Solid Edge part; units mm, degrees
sketch "Sketch1" plane through (0, 0, 0) normal (0, -1, 0) x (1, 0, 0)
  line L0 (-5.8407, 6.1754) -> (-7.1398, 6.9254)
  line L1 (-7.1398, 6.9254) -> (-12.2436, -1.9148)
  line L2 (-12.2436, -1.9148) -> (-9.0862, -3.7377)
  line L3 (-9.0862, -3.7377) -> (-5.1962, 3)
  line L4 (6, 0) -> (6, -2.6279)
  line L5 (13.4768, -2.6279) -> (6, -2.6279)
  line L6 (13.4768, -0.6279) -> (13.4768, -2.6279)
  line L7 (8.4768, -0.6279) -> (13.4768, -0.6279)
  arc A0 (8.4768, -0.6279) -> (-5.8407, 6.1754) centre (0, 0) ccw
  arc A1 (-5.1962, 3) -> (6, 0) centre (0, 0) cw
  dimension "D1" = 5.8407
  dimension "D2" = 13.4768
  dimension "D3" = 8.4768
  dimension "D4" = 6
  dimension "D5" = 13.4768
  dimension "D6" = 12.2436
  dimension "D7" = 9.0862
  dimension "D8" = 7.1398
extrude "Protrusion1" add sketch "Sketch1" against normal blind 2
fillet "Round_1" radius 1 1 edges at (8.4768, 1, -0.6279)
fillet "Round_2" radius 0.5 1 edges at (6, 1, -2.6279)
fillet "Round_3" radius 2 1 edges at (-5.8407, 1, 6.1754)
fillet "Round_4" radius 0.5 1 edges at (-7.1398, 1, 6.9254)
hole "Hole___body" at (-9.6667, 0, -1.0932) direction (0, 1, 0) diameter 2 end up to next
fillet "Round_5" radius 1 2 edges at (-9.0862, 1, -3.7377) (-12.2436, 1, -1.9148)
properties material "ABS Plastic, high impact"
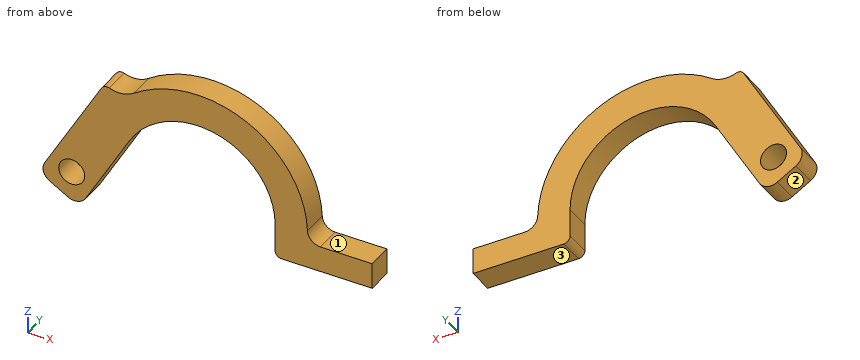
Build history of the part. All positions in model axes, mm. Face numbers are marked on the shaded views. A direction names the side the tool comes from. Round coordinates to 2 decimals unless told otherwise and drop trailing zeros. Loops run counter-clockwise (first coordinate to the right, second up) from the corner with the lowest first, then second, coordinate; pieces in that order, holes last. Notation, with made-up numbers: (-16.5, 64.5) -> (-5.5, 64.5) arc R10 ccw to (-5.5, 72.5) -> close; hole circle Ø4 at (86, -39.5). An arc over 180 degrees is marked (long way). Use CSV: the item, a comma, the result in double quotes. Start each with the question number.
Q1. Saw through at C-C on z = 7.5. Give the cut face in (x, y).
Q2. Which spindle directions (+Z, -Z, +X, -X, +Y, -Y) get a long thin tool onto all of the face, cutting with end or side? Do the marked faces 1, 2 and 3. Say none if no direction does.
Q3. Saw through at B-B on x = -9. Give the cut face in (y, z).
Q4. Saw through at A-A on z = 5.25. Give the cut face in (x, y).
Q5. Drill centre lines: L1, parallel to X at y = 0.9, z = -1; L2, parallel to X at y = 0.6, z = -2; L3, parallel to Z at x = 12, y = 0.55. Where is each one in solid material? Low to high.
Q6. Flat gauge pins, fed straight in: pin 1 Ø2 at (x, z) = (-4.5, -1.5) entering from -Y; pin 2 Ø1 at (x, y) = (8, 0.5) entering from +Z. Where does each tip first touch, or does it go through?
Solutions:
1,outline,"(-4, 0) -> (4, 0) -> (4, 2) -> (-4, 2) -> close"
2,face 1,"+Z, +X, +Y, -Y"
2,face 2,"-Z, -X, +Y, -Y"
2,face 3,"-Z, +X, +Y, -Y"
3,outline,"(0, -3.26) -> (2, -3.26) -> (2, -1.84) -> (0, -1.84) -> close; (0, -0.35) -> (2, -0.35) -> (2, 3.7) -> (0, 3.7) -> close"
4,outline,"(-8.11, 0) -> (-2.9, 0) -> (-2.9, 2) -> (-8.11, 2) -> close; (2.9, 0) -> (6.68, 0) -> (6.68, 2) -> (2.9, 2) -> close"
5,L1,"x = -11.72 to -10.66, -8.67 to -7.51, 6 to 13.48"
5,L2,"x = -11.77 to -10.09, -9.25 to -8.08, 6 to 13.48"
5,L3,"z = -2.63 to -0.63"
6,pin 1,"passes through"
6,pin 2,"stops at z = 4"
